```python
from build123d import *

# Parameters (mm, degrees)
F0_R          = 3.175
F1_DEPTH      = 28.575
F3_R          = 5.0165
F4_DEPTH      = 1.905
F5_R          = 0.254
F6_R          = 0.9525
F7_DEPTH      = 5.0175
F7_DEPTH_BACK = 25.4
F8_R          = 0.508


with BuildPart() as f1:
    # F0 (on Top) → F1 (new body, symmetric)
    with BuildSketch(Plane.XY):
        Circle(F0_R)
    extrude(amount=F1_DEPTH, both=True)

    # F3 (on offset) → F4 (join)
    with BuildSketch(Plane.XY.offset(6.35)):
        Circle(F3_R)
    extrude(amount=F4_DEPTH)

    # F5
    f5_edges = [f1.edges().sort_by_distance(p)[0] for p in [
        (-5.0165, 0, 8.255),
        (-5.0165, 0, 6.35),
    ]]
    fillet(f5_edges, radius=F5_R)

    # F6 (on Right) → F7 (cut, two sides)
    with BuildSketch(Plane.YZ) as f7_sk:
        with Locations((0, -26.035)):
            Circle(F6_R)
    extrude(amount=-F7_DEPTH, mode=Mode.SUBTRACT)
    extrude(f7_sk.sketch, amount=F7_DEPTH_BACK, mode=Mode.SUBTRACT)

    # F8
    f8_edges = [f1.edges().sort_by_distance(p)[0] for p in [
        (-3.175, 0, 28.575),
        (-3.175, 0, -28.575),
    ]]
    fillet(f8_edges, radius=F8_R)


solid = f1.part
```
CAD build for the part. Positions are in the model's coordinates, mm. A direction names the side the tool comes from. Give positions to 0.01 mm unless a question says otherwise; leave off trailing zeros. Order: outer loops, then holes, each group sorted by start corner. A loop starts at its lowest first (then second) coordinate and runs counter-clockwise, first axis right, second up.
(1) Saw through at B-B, the plane z = -6.5. Give the cut face in (x, y) (3 decimals).
(2) Flat gauge pins, fed straight in: pin 1 (2 mm diameter, centred on x = 0, z = 16.5, fed in from +Y) (3 decimals); pin 2 (3 mm diameter, centred on y = 0, z = -26.035, fed in from -X) (3 decimals); pin 3 (6 mm diameter, centred on x = -3.5, z = 13.5, fed in from -Y). Where does each tip first touch, or does it go through?
(3) Tool access for faces 1 (the cylindrical face through (3.03, 0.95, -10.62)), 2 (the flat face through (0, 0, -28.575)), 3 (the cylindrical face through (-0.69, -3.1, 18.3)): list every direction of +Z, -Z, +X, -X, +Y, -Y with a clear straight run to the whole face (end or side of a thin tool).
(4) Drill centre lines: L1, parallel to Z at x = 1.5, y = 0 (1 decimal); L2, parallel to Y at x = 0, z = 15 (3 decimals); L3, parallel to Y at x = 2.75, z = -25.5. Where is each one in solid material? Low to high.
Results found:
1. outline: circle Ø6.35 at (0, 0)
2. pin 1: stops at y = 3.175
2. pin 2: stops at x = -3.175
2. pin 3: stops at y = -3.14
3. face 1: -Z
3. face 2: -Z, +X, -X, +Y, -Y
3. face 3: +Z
4. L1: z = -28.6 to -27, -25.1 to 28.6
4. L2: y = -3.175 to 3.175
4. L3: y = -1.59 to -0.79, 0.79 to 1.59
